```python
from build123d import *

# Parameters (mm, degrees)
SKETCH1_R               = 7.5
BOSS_EXTRUDE1_DEPTH     = 20
BOSS_EXTRUDE2_DEPTH     = 100
CUT_EXTRUDE1_DEPTH      = 50
SKETCH4_R               = 10
CUT_EXTRUDE2_DEPTH      = 30
CUT_EXTRUDE2_DEPTH_BACK = 119


with BuildPart() as part:
    # Sketch1 → Boss-Extrude1 (new body)
    with BuildSketch(Plane(origin=(0, 0, 0), x_dir=(1, 0, 0), z_dir=(0, 1, 0))):
        with BuildLine():
            Line((-49.860018769, -23.434965581), (11.985981198, -37.004254746))
            ThreePointArc((11.985981198, -37.004254746), (21.139981231, -38.434965581), (30.293981265, -37.004254746))
            Line((30.293981265, -37.004254746), (89.131173769, -23.130103473))
            ThreePointArc((89.131173769, -23.130103473), (107.063571087, -9.947071997), (92.139981231, 6.565034419))
            Line((92.139981231, 6.565034419), (30.293981265, 20.134323584))
            ThreePointArc((30.293981265, 20.134323584), (21.139981231, 21.565034419), (11.985981198, 20.134323584))
            Line((11.985981198, 20.134323584), (-49.860018769, 6.565034419))
            ThreePointArc((-49.860018769, 6.565034419), (-64.860018769, -8.434965581), (-49.860018769, -23.434965581))
        make_face()
        with Locations((-49.860018769, -8.434965581)):
            Circle(SKETCH1_R, mode=Mode.SUBTRACT)
        with Locations((92.139981231, -8.434965581)):
            Circle(SKETCH1_R, mode=Mode.SUBTRACT)
    extrude(amount=BOSS_EXTRUDE1_DEPTH)

    # Sketch2 → Boss-Extrude2 (add)
    with BuildSketch(Plane(origin=(0, 0, 0), x_dir=(1, 0, 0), z_dir=(0, 1, 0))):
        with BuildLine():
            Line((-7.907393865, -0.934965581), (50.187356328, -0.934965581))
            ThreePointArc((50.187356328, -0.934965581), (21.139981231, 21.565034419), (-7.907393865, -0.934965581))
        make_face()
        with BuildLine():
            Line((50.187356328, -15.934965581), (-7.907393865, -15.934965581))
            ThreePointArc((-7.907393865, -15.934965581), (21.139981231, -38.434965581), (50.187356328, -15.934965581))
        make_face()
    extrude(amount=BOSS_EXTRUDE2_DEPTH)

    # Sketch3 → Cut-Extrude1 (cut)
    with BuildSketch(Plane(origin=(0, 100, 0), x_dir=(1, 0, 0), z_dir=(0, 1, 0))):
        with BuildLine():
            Line((-2.476750126, -26.934965581), (44.756712589, -26.934965581))
            ThreePointArc((44.756712589, -26.934965581), (21.139981231, -38.434965581), (-2.476750126, -26.934965581))
        make_face()
        with BuildLine():
            Line((44.756712589, 10.065034419), (-2.476750126, 10.065034419))
            ThreePointArc((-2.476750126, 10.065034419), (21.139981231, 21.565034419), (44.756712589, 10.065034419))
        make_face()
    extrude(amount=-CUT_EXTRUDE1_DEPTH, mode=Mode.SUBTRACT)

    # Sketch4 → Cut-Extrude2 (cut, two sides)
    with BuildSketch(Plane.XY.offset(26.934965581)) as cut_extrude2_sk:
        with Locations((21.139981231, 76)):
            Circle(SKETCH4_R)
    extrude(amount=CUT_EXTRUDE2_DEPTH, mode=Mode.SUBTRACT)
    extrude(cut_extrude2_sk.sketch, amount=-CUT_EXTRUDE2_DEPTH_BACK, mode=Mode.SUBTRACT)


solid = part.part
```
Geometry check sheet. Reference: the model listing, model coordinates, mm. A direction names the side the tool comes from. Round coordinates to 2 decimals unless told otherwise and drop trailing zeros. Write each loop counter-clockwise with the first axis right and the second up, starting at its lowest first coordinate (ties: lowest second). Pieces come first, ordered by that corner, then holes. Notation, with made-up numbers: (2.5, -32.5) -> (11.5, -32.5) arc R26 ccw to (11.5, -13.5) -> close; hole circle Ø8 at (38, 70.25). An arc over 180 degrees is marked (long way). Put each result on its own line as item: value.
1) Cross-section at A-A, the plane y = 76. Enter the section's corners in (x, z).
Recorded:
outline: (-7.91, 0.93) arc R30 ccw to (-2.48, -10.07) -> (11.14, -10.07) -> (11.14, 0.93) -> close; (-7.91, 15.93) -> (11.14, 15.93) -> (11.14, 26.93) -> (-2.48, 26.93) arc R30 ccw to start; (31.14, -10.07) -> (44.76, -10.07) arc R30 ccw to (50.19, 0.93) -> (31.14, 0.93) -> close; (31.14, 15.93) -> (50.19, 15.93) arc R30 ccw to (44.76, 26.93) -> (31.14, 26.93) -> close
2) Cross-section at D-D, the plane x = 41.5. Enter the section's corners in (y, z).
Recorded:
outline: (0, -17.68) -> (20, -17.68) -> (20, -13.6) -> (50, -13.6) -> (50, -10.07) -> (100, -10.07) -> (100, 0.93) -> (20, 0.93) -> (20, 15.93) -> (100, 15.93) -> (100, 26.93) -> (50, 26.93) -> (50, 30.47) -> (20, 30.47) -> (20, 34.36) -> (0, 34.36) -> close
3) Thickness scan on probe 1 along Z at (x, y) = (36, 88); probe 2 along Y at (x, z) = (21, 18); probe 3 along Y at (x, z) = (62, 18). Record the ranges inside material, lowest first. Write a range as from..to.
Recorded:
probe 1: z = -10.07..0.93, 15.93..26.93
probe 2: y = 0..66, 86..100
probe 3: y = 0..20
4) Cross-section at B-B, the plane y = 92. Enter the section's corners in (x, z).
Recorded:
outline: (-7.91, 0.93) arc R30 ccw to (-2.48, -10.07) -> (44.76, -10.07) arc R30 ccw to (50.19, 0.93) -> close; (-7.91, 15.93) -> (50.19, 15.93) arc R30 ccw to (44.76, 26.93) -> (-2.48, 26.93) arc R30 ccw to start
5) Depth check by flat-ended pin: P1, Ø17.5, axis at x = 32, y = 44, coming from the -Z side; P2, Ø1.5, axis at x = 47.5, y = 25, coming from the +Z side; P3, Ø16, axis at x = 21.14, y = 76, coming from the -Z side; P4, Ø14, axis at x = 19.5, y = 72.5, coming from the +Z side. Enter the tip coordinate at first touch or a pass-through.
Recorded:
P1: stops at z = -21.49
P2: stops at z = 24.06
P3: passes through
P4: stops at z = 26.93
6) Release check for a two-part mould opening along X. For faces 6 (the face through (19.838, 85.915, 21.512)), 7 (the face through (61.65, 9.86, -13.255)), 8 (the face through (19.838, 85.915, -4.488)), 9 (the face through (21, 59, 0.935)) record: pulls with the +X half, pulls with the -X half, needs draft (parallel to the pull), parting line crosses it, or undercut.
Recorded:
face 6: undercut
face 7: pulls with the +X half
face 8: undercut
face 9: needs draft
7) Cross-section at C-C, the plane z = 12. Enter the section's corners in (x, y).
Recorded:
outline: (-64.43, 0) -> (-56.46, 0) -> (-56.46, 20) -> (-64.43, 20) -> close; (-43.26, 0) -> (85.54, 0) -> (85.54, 20) -> (-43.26, 20) -> close; (98.74, 0) -> (106.71, 0) -> (106.71, 20) -> (98.74, 20) -> close
8) Access from +Z, -Z, +X, -X, +Y, -Y to the whole of each face (thin tool, end or side, straight path). Record for faces 1 (the face through (22, 59, 15.935)), 2 (the face through (21, 50, 31)), 3 (the face through (20.59, 38.19, 38.43)), 4 (the face through (11, 75, -10.065)), 5 (the face through (-57.353, 9.86, 8.105)).
Recorded:
face 1: +X, -X, +Y
face 2: +Z, +X, -X, +Y
face 3: +Z, +Y
face 4: -Z, +X, -X, +Y
face 5: +Y, -Y
